Source: CAD feature listing. Evaluate the final solid. Frame: model axes, mm. A direction names the side the tool comes from. Give positions to 0.01 mm unless a question says otherwise; leave off trailing zeros. Loops run counter-clockwise (first coordinate to the right, second up) from the corner with the lowest first, then second, coordinate; pieces in that order, holes last. Notation, with made-up numbers: M -31,58 L 3,58 A15 cw 3,64 Z; hole C 83,52.25 d7. An arc over 180 degrees is marked long. Answer in a Markdown table with one row per item.
```python
from build123d import *


with BuildPart() as f1:
    # F0 (on Front) → F1 (revolve)
    with BuildSketch(Plane.XZ):
        with BuildLine():
            Line((0, 166.624), (0, 0))
            Line((0, 0), (0, -352.298))
            Line((0, -352.298), (134.239, -352.298))
            Line((134.239, -352.298), (134.239, -430.022))
            Line((134.239, -430.022), (224.604496, -430.022))
            ThreePointArc((224.604496, -430.022), (215.021889, -401.859149), (195.503543, -379.409055))
            ThreePointArc((195.503543, -379.409055), (176.878926, -344.15539), (190.957997, -306.852883))
            ThreePointArc((190.957997, -306.852883), (220.997872, -235.94093), (193.391806, -164.046534))
            ThreePointArc((193.391806, -164.046534), (136.113903, 34.381675), (262.333799, 197.853539))
            ThreePointArc((262.333799, 197.853539), (293.322046, 226.516887), (302.514, 267.716))
            Line((302.514, 267.716), (134.239, 267.716))
            Line((134.239, 267.716), (134.239, 166.624))
            Line((134.239, 166.624), (0, 166.624))
        make_face()
    revolve(axis=Axis((0, 0, -176.149), (0, 0, -1)))


solid = f1.part
```
Q1. Section query D-D (z = 223). Output: boundary loops of the cut face in (x, y), plus the area to 3 significant figures.
Values follow:
| item | result |
|---|---|
| outline | C 0,0 d582.32; hole C 0,0 d268.48 |
| area | 210,000 mm^2 |
Q2. Ray query, probe 1 along Z at (x, y) = (154, -93.5); probe 2 along Z at (x, y) = (184, -102.5); probe 3 along Y at (x, z) = (0, 244). Return the intervals inside material, ascending. Write a range as from..to.
Values follow:
| item | result |
|---|---|
| probe 1 | -430.02..-358.91, -323.34..-148.52, 131.82..267.72 |
| probe 2 | -430.02..-395.06, -279.24..-189.14, 163.99..267.72 |
| probe 3 | -300.47..-134.24, 134.24..300.47 |
Q3. Mould query, pull axis Y, two halves, no side actions, for faces 1 (the flat face through (63, 130, 267.716)), 2 (the flat face through (-2, -2, 166.624)). Classes: +Y half, -Y half, draft (parallel to the pull), parting line (faces both ways), or undercut.
Values follow:
| item | result |
|---|---|
| face 1 | draft |
| face 2 | undercut |
Q4. Section query A-A (y = 0). Output: boundary loops of the cut face in (x, z), plus the area to 3 significant figures.
Values follow:
| item | result |
|---|---|
| outline | M -302.51,267.72 A70.87 ccw -262.33,197.85 A228.35 cw -193.39,-164.05 A102.87 ccw -190.96,-306.85 A48.51 cw -195.5,-379.41 A77.22 ccw -224.6,-430.02 L -134.24,-430.02 L -134.24,-352.3 L 134.24,-352.3 L 134.24,-430.02 L 224.6,-430.02 A77.22 ccw 195.5,-379.41 A48.51 cw 190.96,-306.85 A102.87 ccw 193.39,-164.05 A228.35 cw 262.33,197.85 A70.87 ccw 302.51,267.72 L 134.24,267.72 L 134.24,166.62 L -134.24,166.62 L -134.24,267.72 Z |
| area | 218,000 mm^2 |
Q5. Reachability of faces 3 (the cylindrical face through (128.04, -40.32, -391.7)), 4 (the cylindrical face through (128.04, -40.32, 216.46)), 5 (the flat face through (-97, 97, -430.022)) from +Z, -Z, +X, -X, +Y, -Y: full face, straight path, thin tool, end or side. Return the list, or none.
Values follow:
| item | result |
|---|---|
| face 3 | -Z |
| face 4 | +Z |
| face 5 | -Z, +X, -X, +Y, -Y |
Q6. Contact query for flat-ended pins moving along their axis: pin 1 Ø8 at (y, z) = (145, -337) entering from -X; pin 2 Ø8 at (x, z) = (54.5, -218) entering from +Y; pin 3 Ø6 at (y, z) = (136.5, -345.5) entering from +X. Output: stop coordinate, or through.
Values follow:
| item | result |
|---|---|
| pin 1 | x = -106.96 |
| pin 2 | y = 214.03 |
| pin 3 | x = 116.22 |
Q7. Section query B-B (y = -210). Give the number of separate pieces and of enclosed holes in the cut face, plus the area to 3 significant figures.
Values follow:
| item | result |
|---|---|
| separate pieces | 3 |
| enclosed holes | 0 |
| area | 49,300 mm^2 |
